Geometry check sheet. Reference: drawing and pictorial views, mm from the part's lowest x, y, z. Coordinates: 2 decimals unless noted, no trailing zeros. Loops run counter-clockwise (first coordinate to the right, second up) from the corner with the lowest first, then second, coordinate; pieces in that order, holes last. Notation, with made-up numbers: (-11.5, 3.5) -> (-4.5, 3.5) arc R8 cw to (-4.5, 17.5) -> close; hole circle Ø4 at (37.25, 53). An arc over 180 degrees is marked (long way). Answer as a JSON object with one key per item and string values. Group by question number.
Q1. Cross-section at A-A on z = 8.5. Record the boundary of the cut face in (x, y).
Q2. Gauge pin test, flat end, axial feed: pin 1 Ø1.5 at (x, y) = (2, 1) entering from -Z. Record the tip position at first contact, or that the pin passes through.
Q3. Scan lines: L1, parallel to Z at x = 2.05, y = 2.4; L2, parallel to Y at x = 1.4, z = 0.5; L3, parallel to Z at x = 1.2, y = 2.85 (1 decimal). Record each from-to range of solid material in increasing order.
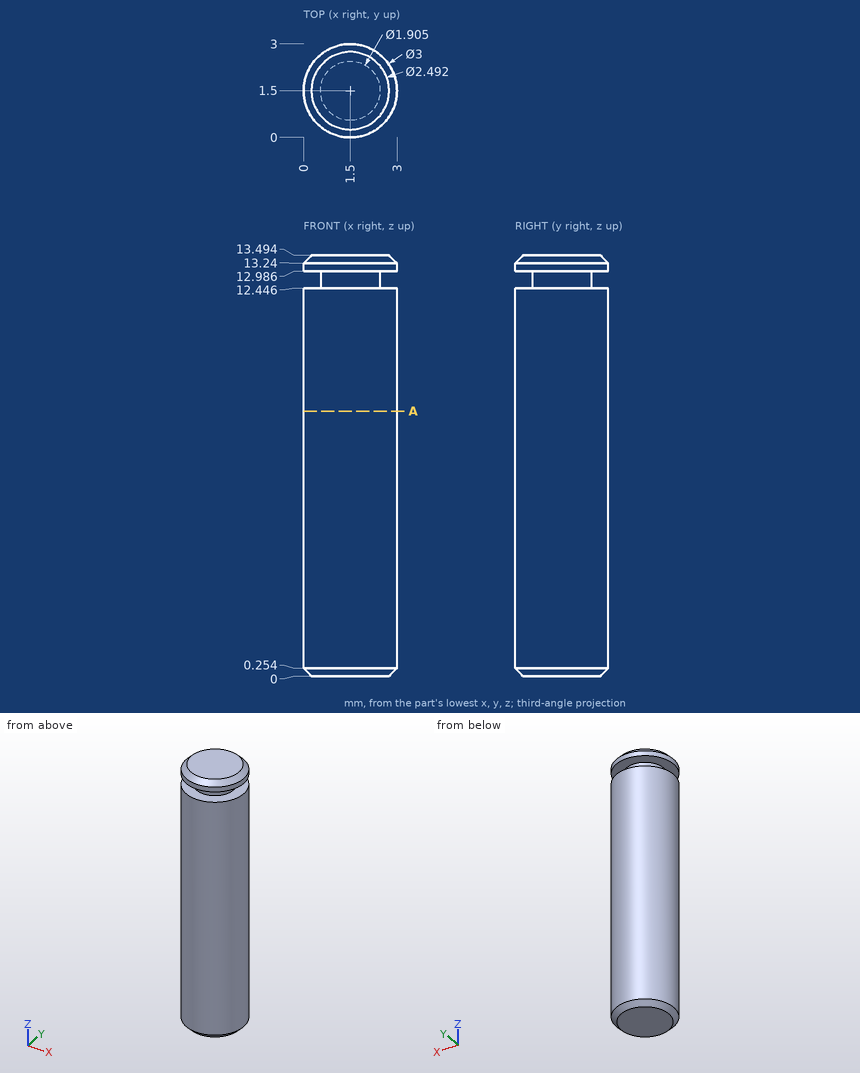
Computed values:
{
 "1": {"outline": "circle Ø3 at (1.5, 1.5)"},
 "2": {"pin 1": "stops at z = 0"},
 "3": {"L1": "z = 0 to 12.45, 12.99 to 13.49", "L2": "y = 0 to 3", "L3": "z = 0.1 to 12.4, 13 to 13.4"}
}
